Can you work these out from the model? Positions are in its coordinate system, mm. Face numbers are marked on the shaded views. A direction names the side the tool comes from. Give positions to 0.01 mm unless a question says otherwise; leave off trailing zeros. Order: outer loops, then holes, each group sorted by start corner. A loop starts at its lowest first (then second) coordinate and runs counter-clockwise, first axis right, second up. Notation, with made-up numbers: M 24.25,0 L 81.25,0 A22 ccw 81.25,39 Z; hole C -10.75,-17 d10. An arc over 180 degrees is marked long. Answer as a JSON object with one key per item and string values.
```python
from build123d import *

# Parameters (mm, degrees)
F1_DEPTH = 145
F3_DEPTH = 108.001
F4_W     = 40
F4_H     = 25
F4_W_2   = 14
F4_H_2   = 10
F5_DEPTH = 5.001
F7_DEPTH = 108.001


with BuildPart() as f1:
    # F0 (on Front) → F1 (new body)
    with BuildSketch(Plane.XZ):
        Polygon((-54, 20), (-54, 0), (-31, 0), (-31, -1.15), (-33.5, -1.15), (-33.5, -2), (-25.5, -2), (-25.5, 0), (25.5, 0), (25.5, -2), (33.5, -2), (33.5, -1.15), (31, -1.15), (31, 0), (54, 0), (54, 20), (52, 20), (52, 3), (0, 3), (-52, 3), (-52, 20), align=None)
    extrude(amount=F1_DEPTH)

    # F2 (on face) → F3 (cut, through all)
    with BuildSketch(Plane.YZ.offset(54)):
        with BuildLine():
            Line((-109, 11.15), (-124, 11.15))
            ThreePointArc((-124, 11.15), (-125.8, 9.35), (-124, 7.55))
            Line((-124, 7.55), (-109, 7.55))
            ThreePointArc((-109, 7.55), (-107.2, 9.35), (-109, 11.15))
        make_face()
        with BuildLine():
            ThreePointArc((-22, 11.15), (-23.8, 9.35), (-22, 7.55))
            Line((-22, 7.55), (-7, 7.55))
            ThreePointArc((-7, 7.55), (-5.2, 9.35), (-7, 11.15))
            Line((-7, 11.15), (-22, 11.15))
        make_face()
    extrude(amount=-F3_DEPTH, mode=Mode.SUBTRACT)

    # F4 (on face) → F5 (cut, through all)
    with BuildSketch(Plane.XY.offset(3)):
        with Locations((0, -27.5)):
            Rectangle(F4_W, F4_H)
        with Locations((-40, -15)):
            Rectangle(F4_W_2, F4_H_2)
        with Locations((-40, -43.5)):
            Rectangle(F4_W_2, F4_H_2)
        with Locations((-40, -72)):
            Rectangle(F4_W_2, F4_H_2)
        with Locations((-40, -100.5)):
            Rectangle(F4_W_2, F4_H_2)
        with Locations((-40, -129)):
            Rectangle(F4_W_2, F4_H_2)
        with Locations((42, -15)):
            Rectangle(F4_W_2, F4_H_2)
        with Locations((42, -43.5)):
            Rectangle(F4_W_2, F4_H_2)
        with Locations((42, -72)):
            Rectangle(F4_W_2, F4_H_2)
        with Locations((42, -100.5)):
            Rectangle(F4_W_2, F4_H_2)
        with Locations((42, -129)):
            Rectangle(F4_W_2, F4_H_2)
        with Locations((0, -72.5)):
            Rectangle(F4_W, F4_H)
        with Locations((0, -117.5)):
            Rectangle(F4_W, F4_H)
    extrude(amount=-F5_DEPTH, mode=Mode.SUBTRACT)

    # F6 (on face) → F7 (cut, through all)
    with BuildSketch(Plane(origin=(-54, 0, 0), x_dir=(0, -1, 0), z_dir=(-1, 0, 0))):
        with BuildLine():
            Line((95, 20), (50, 20))
            Line((50, 20), (50, 13))
            ThreePointArc((50, 13), (51.464466, 9.464466), (55, 8))
            Line((55, 8), (90, 8))
            ThreePointArc((90, 8), (93.535534, 9.464466), (95, 13))
            Line((95, 13), (95, 20))
        make_face()
    extrude(amount=-F7_DEPTH, mode=Mode.SUBTRACT)


solid = f1.part
```
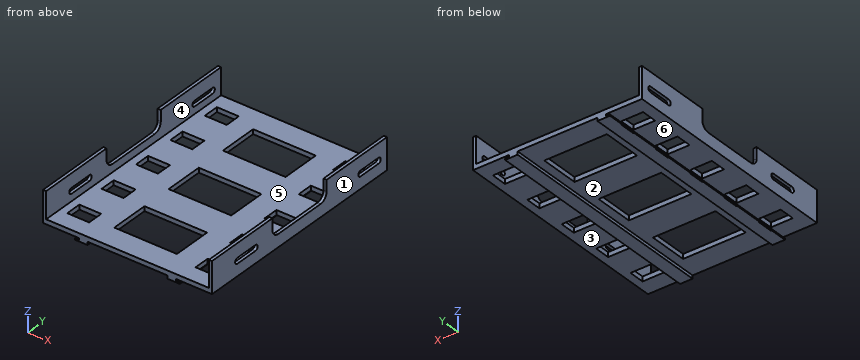
1) I want a section at B-B on x = 39.5. Write out the boundary of the cut face in (y, z), and give its area (3 significant figures).
Results found:
{"outline": "M -145,0 L -134,0 L -134,3 L -145,3 Z; M -124,0 L -105.5,0 L -105.5,3 L -124,3 Z; M -95.5,0 L -77,0 L -77,3 L -95.5,3 Z; M -67,0 L -48.5,0 L -48.5,3 L -67,3 Z; M -38.5,0 L -20,0 L -20,3 L -38.5,3 Z; M -10,0 L 0,0 L 0,3 L -10,3 Z", "area": "285 mm²"}
2) I want a section at D-D on y = -64.5. Write out the boundary of the cut face in (x, z).
Results found:
{"outline": "M -54,0 L -31,0 L -31,-1.15 L -33.5,-1.15 L -33.5,-2 L -25.5,-2 L -25.5,0 L -20,0 L -20,3 L -52,3 L -52,8 L -54,8 Z; M 20,0 L 25.5,0 L 25.5,-2 L 33.5,-2 L 33.5,-1.15 L 31,-1.15 L 31,0 L 54,0 L 54,8 L 52,8 L 52,3 L 20,3 Z"}
3) I want a section at C-C on z = 17.5. Write out the boundary of the cut face in (x, y).
Results found:
{"outline": "M -54,-145 L -52,-145 L -52,-95 L -54,-95 Z; M -54,-50 L -52,-50 L -52,0 L -54,0 Z; M 52,-145 L 54,-145 L 54,-95 L 52,-95 Z; M 52,-50 L 54,-50 L 54,0 L 52,0 Z"}
4) I need wall thicknesses on L1, parallel to Y at x = 0, z = 1.25; L2, parallel to X at y = -16.5, z = 2.75; L3, parallel to Y at x = 44, z = 2.5. Which ranges of each line are inside material? Lowest first, please.
Results found:
{"L1": "y = -145 to -130, -105 to -85, -60 to -40, -15 to 0", "L2": "x = -54 to -47, -33 to -20, 20 to 35, 49 to 54", "L3": "y = -145 to -134, -124 to -105.5, -95.5 to -77, -67 to -48.5, -38.5 to -20, -10 to 0"}
5) I want a section at A-A on y = -98.5. Write out the boundary of the cut face in (x, z).
Results found:
{"outline": "M -54,0 L -47,0 L -47,3 L -52,3 L -52,20 L -54,20 Z; M -33,-2 L -25.5,-2 L -25.5,0 L 25.5,0 L 25.5,-2 L 33.5,-2 L 33.5,-1.15 L 31,-1.15 L 31,0 L 35,0 L 35,3 L -33,3 L -33,0 L -31,0 L -31,-1.15 L -33,-1.15 Z; M 49,0 L 54,0 L 54,20 L 52,20 L 52,3 L 49,3 Z"}
6) I'm going to push flat-ended pins straight in: pin 1 Ø5 at (x, y) = (42.5, -40) entering from +Z; pin 2 Ø1.3 at (y, z) = (-76.5, -0.5) entering from +X; pin 3 Ø0.6 at (y, z) = (-68.5, -1.5) entering from -X; pin 4 Ø0.9 at (y, z) = (-141.5, -1.5) entering from -X. Where does each tip first touch, or does it pass through?
Results found:
{"pin 1": "stops at z = 3", "pin 2": "stops at x = 54", "pin 3": "stops at x = -33", "pin 4": "stops at x = -33.5"}
7) For the marked faces 1, 2 and 3, which set-ups out of +Z, -Z, +X, -X, +Y, -Y let a thin tool reach every point of the face, with its end or its side?
Results found:
{"face 1": "+Z, -Z, +X, +Y, -Y", "face 2": "-Z, +Y, -Y", "face 3": "+X, +Y, -Y"}
8) Thinking about a two-plate mould opening in Z: for the marked faces 4, 5 and 6, which applies, pulls with the +Z half, pulls with the -Z half, needs draft (parallel to the pull), parting line crosses it, or undercut?
Results found:
{"face 4": "needs draft", "face 5": "pulls with the +Z half", "face 6": "undercut"}
